from build123d import *

# Parameters (mm, degrees)
SKETCH1_R           = 2.838382548
BOSS_EXTRUDE2_DEPTH = 12.7
FILLET5_R           = 33.02
FILLET7_R           = 2.54


with BuildPart() as part:
    # Sketch1 → Boss-Extrude2 (new body)
    with BuildSketch(Plane.XY):
        with BuildLine():
            Line((-21.603638559, 84.96960614), (29.87982891, 77.564224626))
            Line((29.87982891, 77.564224626), (113.413965473, 47.151661477))
            Line((113.413965473, 47.151661477), (109.035804568, 35.126174209))
            Line((109.035804568, 35.126174209), (95.280304394, 0.145728286))
            Line((95.280304394, 0.145728286), (81.56676708, -34.728005444))
            Line((81.56676708, -34.728005444), (69.33354083, -37.004919145))
            Line((69.33354083, -37.004919145), (61.026465875, -17.204201513))
            ThreePointArc((61.026465875, -17.204201513), (76.334091657, 9.884016708), (53.926809391, 31.471250781))
            ThreePointArc((53.926809391, 31.471250781), (47.534060902, 31.352091343), (41.37361205, 29.640278808))
            Line((41.37361205, 29.640278808), (1.321326785, 44.395112668))
            Line((1.321326785, 44.395112668), (-32.231275521, 69.307770201))
            Line((-32.231275521, 69.307770201), (-21.603638559, 84.96960614))
        make_face()
        with Locations((20.390142766, 51.502972215)):
            Circle(SKETCH1_R, mode=Mode.SUBTRACT)
        with BuildLine():
            Line((24.516957739, 66.398380962), (-13.583042261, 71.878684632))
            ThreePointArc((-13.583042261, 71.878684632), (-16.074090815, 75.206755234), (-12.746020212, 77.697803788))
            Line((-12.746020212, 77.697803788), (25.353979788, 72.217500118))
            ThreePointArc((25.353979788, 72.217500118), (27.845028342, 68.889429516), (24.516957739, 66.398380962))
        make_face(mode=Mode.SUBTRACT)
    extrude(amount=BOSS_EXTRUDE2_DEPTH)

    # Fillet5
    fillet5_edges = [part.edges().sort_by_distance(p)[0] for p in [
        (113.413965473, 47.151661477, 6.35),
    ]]
    fillet(fillet5_edges, radius=FILLET5_R)

    # Fillet7
    fillet7_edges = [part.edges().sort_by_distance(p)[0] for p in [
        (81.56676708, -34.728005444, 6.35),
        (69.33354083, -37.004919145, 6.35),
    ]]
    fillet(fillet7_edges, radius=FILLET7_R)


solid = part.part
The listing builds one solid part. Answer for the finished solid, in the listing's coordinates (mm). A direction names the side the tool comes from. Round coordinates to 2 decimals unless told otherwise and drop trailing zeros. Order: outer loops, then holes, each group sorted by start corner. A loop starts at its lowest first (then second) coordinate and runs counter-clockwise, first axis right, second up. Notation, with made-up numbers: M -36,28 L 19,28 A17 ccw 19,37 Z; hole C 62,55.25 d10. An arc over 180 degrees is marked long. Answer in a Markdown table with one row per item. Add a question column.
1) Consider line 1 along Y through (x, z) = (23, 10.5); line 2 along Y through (x, z) = (1.5, 10.75); line 3 along Y through (x, z) = (27.5, 9). Determine where each line is inside the solid, lowest interval first. Write a range as from..to.
2) Determine the mould class of faces 3 (the face through (55.52, 68.23, 6.26)), 4 (the face through (27.854, 68.954, 6.261)), 5 (the face through (69.7, -36.38, 6.44)) for opening direction Y: pulls with the +Y half, pulls with the -Y half, needs draft (parallel to the pull), parting line crosses it, or undercut.
3) Flat-ended cylindrical pins translate along their axes: pin 1 Ø2 at (y, z) = (22.5, 6) entering from +X; pin 2 Ø1.5 at (x, z) = (39.5, 7) entering from +Y; pin 3 Ø5 at (y, z) = (-22.5, 7.5) entering from -X. Find the tip coordinate at first contact, or state that the pin passes through.
4) Which of the six approach directions +Z, -Z, +X, -X, +Y, -Y give full straight-line access (tool end or side, diameter ignored) to faces 1 (the face through (-26.99, 77.03, 6.26)), 2 (the face through (6, 75, 6))?
5) The part is cut by section A-A on x = 15. Determine the outline of the cut face in (y, z), plus the area to 3 significant figures.
6) The part is cut by section C-C on z = 9.25. Count the separate pieces of the cut face and the enclosed holes in it, plus the area to 3 significant figures.
7) The part is cut by section D-D on y = 4. Determine the outline of the cut face in (x, z), plus the area to 3 significant figures.
8) The part is cut by section B-B on x = -7. Determine the outline of the cut face in (y, z).
Findings below:
| question | item | result |
|---|---|---|
| 1 | line 1 | y = 36.41..50.39, 52.62..66.62, 72.56..78.55 |
| 1 | line 2 | y = 44.33..69.71, 75.65..81.65 |
| 1 | line 3 | y = 34.75..67.87, 70.74..77.91 |
| 2 | face 3 | pulls with the +Y half |
| 2 | face 4 | undercut |
| 2 | face 5 | pulls with the -Y half |
| 3 | pin 1 | stops at x = 103.36 |
| 3 | pin 2 | stops at y = 74.33 |
| 3 | pin 3 | stops at x = 62.2 |
| 4 | face 1 | +Z, -Z, -X, +Y |
| 4 | face 2 | +Z, -Z |
| 5 | outline | M 39.36,0 L 67.77,0 L 67.77,12.7 L 39.36,12.7 Z; M 73.71,0 L 79.7,0 L 79.7,12.7 L 73.71,12.7 Z |
| 5 | area | 437 mm² |
| 6 | separate pieces | 1 |
| 6 | enclosed holes | 2 |
| 6 | area | 5,640 mm² |
| 7 | outline | M 76.5,0 L 96.8,0 L 96.8,12.7 L 76.5,12.7 Z |
| 7 | area | 258 mm² |
| 8 | outline | M 50.57,0 L 70.93,0 L 70.93,12.7 L 50.57,12.7 Z; M 76.87,0 L 82.87,0 L 82.87,12.7 L 76.87,12.7 Z |
